Check sheet for the drawn part. Datum: minimum x, y, z corner. Units: mm. Round coordinates to 2 decimals unless told otherwise and drop trailing zeros. Loops run counter-clockwise (first coordinate to the right, second up) from the corner with the lowest first, then second, coordinate; pieces in that order, holes last. Notation, with made-up numbers: (51.5, 0.25) - (103.5, 0.25) arc R38 cw to (103.5, 39.25) - close; hole circle Ø9 at (63, 37). An arc over 180 degrees is marked (long way). Use CSV: the item, a comma, the result in double quotes.
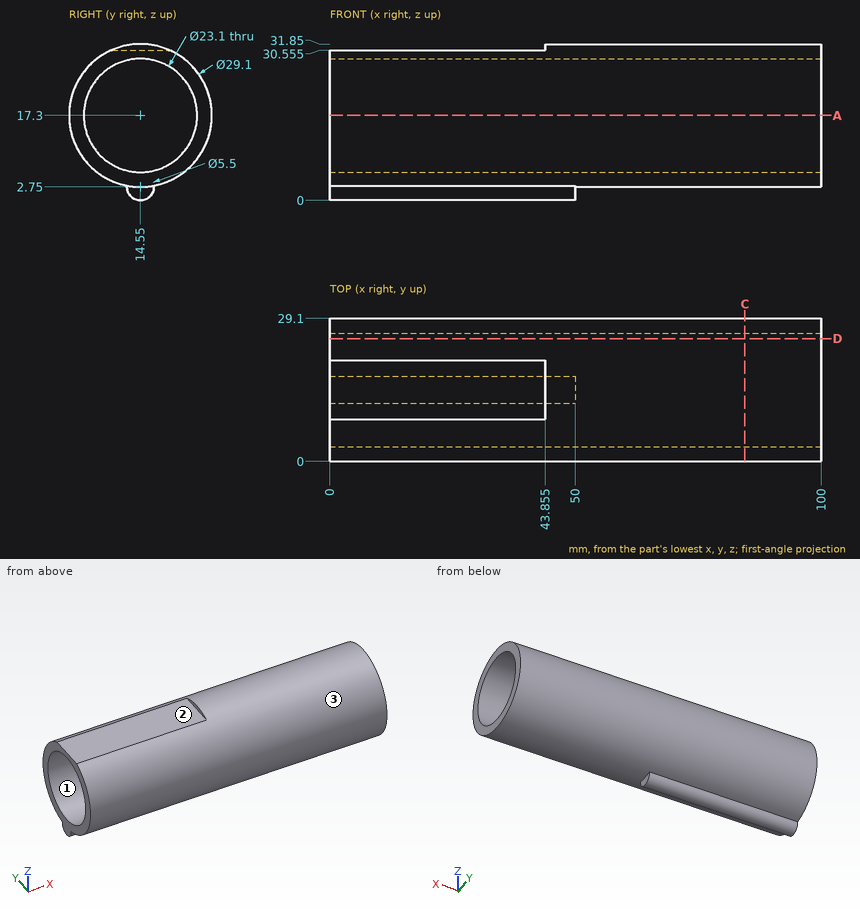
1) Gauge pin test, flat ends, axial feed: pin 1 Ø8 at (x, z) = (22, 3.5) entering from -Y (1 decimal); pin 2 Ø1.5 at (x, z) = (52, 4) entering from -Y; pin 3 Ø4 at (x, y) = (75.5, 18.5) entering from -Z. Record the tip position at first contact, or that the pin passes through.
Returned:
pin 1,"stops at y = 3.8"
pin 2,"stops at y = 7.19"
pin 3,"stops at z = 2.88"
2) Cross-section at A-A, the plane z = 17.3. Record the cut outline in (x, y), then the cut area to 3 significant figures.
Returned:
outline,"(0, 0) - (100, 0) - (100, 3) - (0, 3) - close; (0, 26.1) - (100, 26.1) - (100, 29.1) - (0, 29.1) - close"
area,"600 mm²"
3) Thickness scan on probe 1 along Z at (x, y) = (57, 14.55); probe 2 along Y at (x, z) = (55, 17.3); probe 3 along Z at (x, y) = (48, 21). Record the ranges inside material, lowest first. Write a range as [from, to].
Returned:
probe 1,"z = [2.75, 5.75], [28.85, 31.85]"
probe 2,"y = [0, 3], [26.1, 29.1]"
probe 3,"z = [4.26, 7.72], [26.88, 30.34]"
4) Mould release check, pull along Y, two halves, no side actions. Record for the marked faces 1, 2 and 3: +Y half, -Y half, draft (parallel to the pull), parting line (faces both ways), or undercut.
Returned:
face 1,"undercut"
face 2,"draft"
face 3,"parting line"
5) Cross-section at C-C, the plane x = 84.5. Record the cut outline in (y, z), then the cut area to 3 significant figures.
Returned:
outline,"circle Ø29.1 at (14.55, 17.3); hole circle Ø23.1 at (14.55, 17.3)"
area,"246 mm²"
6) Cross-section at D-D, the plane y = 25. Record the cut outline in (x, z), then the cut area to 3 significant figures.
Returned:
outline,"(0, 7.18) - (100, 7.18) - (100, 12.38) - (0, 12.38) - close; (0, 22.22) - (100, 22.22) - (100, 27.42) - (0, 27.42) - close"
area,"1,040 mm²"
